Here's how the part is built. I have some questions about the finished solid (model axes, mm). Face numbers are marked on the shaded views. Give positions to 0.01 mm unless a question says otherwise; leave off trailing zeros. Put each result on its own line as item: value. Start each with the question number.
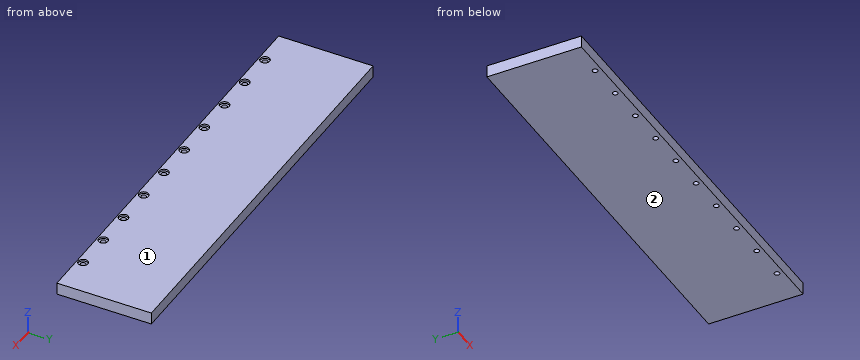
from build123d import *

# Parameters (mm, degrees)
SKETCH1_W                        = 220
SKETCH1_H                        = 50
BOSS_EXTRUDE1_DEPTH              = 3.175
CBORE_FOR_M2_5_SHCS1_D           = 2.7
CBORE_FOR_M2_5_SHCS1_DEPTH       = 15
CBORE_FOR_M2_5_SHCS1_CBORE_D     = 5
CBORE_FOR_M2_5_SHCS1_CBORE_DEPTH = 1
CBORE_FOR_M2_5_SHCS1_TIP         = 0.811161836


with BuildPart() as part:
    # Sketch1 → Boss-Extrude1 (new, symmetric)
    with BuildSketch(Plane.XY):
        Rectangle(SKETCH1_W, SKETCH1_H)
    extrude(amount=BOSS_EXTRUDE1_DEPTH, both=True)

    # CBORE for M2.5 SHCS1
    with Locations(Plane.XY.offset(3.175)):
        with Locations((89.95, -21.825), (69.9, -21.825), (49.85, -21.825), (29.8, -21.825), (9.75, -21.825), (-10.3, -21.825), (-30.35, -21.825), (-50.4, -21.825), (-70.45, -21.825), (-90.5, -21.825)):
            CounterBoreHole(CBORE_FOR_M2_5_SHCS1_D / 2, CBORE_FOR_M2_5_SHCS1_CBORE_D / 2, CBORE_FOR_M2_5_SHCS1_CBORE_DEPTH, depth=CBORE_FOR_M2_5_SHCS1_DEPTH)
            with Locations((0, 0, -(CBORE_FOR_M2_5_SHCS1_DEPTH + CBORE_FOR_M2_5_SHCS1_TIP / 2))):  # 118° drill point
                Cone(0, CBORE_FOR_M2_5_SHCS1_D / 2, CBORE_FOR_M2_5_SHCS1_TIP, mode=Mode.SUBTRACT)


solid = part.part
1) I'm going to push a flat-ended pin straight in: P1, Ø4.5, axis at x = -30.35, y = -21.825, coming from the +Z side (3 decimals). Where does the tip first touch, or does it pass through?
2) Thinking about a two-plate mould opening in Z: for the marked faces 1 and 2, which applies, pulls with the +Z half, pulls with the -Z half, needs draft (parallel to the pull), parting line crosses it, or undercut?
3) I need wall thicknesses on line 1 (Y direction, x = -50.4, z = 2.7) (3 decimals); line 2 (Y direction, x = 29.8, z = -0.9) (3 decimals). Which ranges of each line are inside material? Lowest first, please.
Ans:
1. P1: stops at z = 2.175
2. face 1: pulls with the +Z half
2. face 2: pulls with the -Z half
3. line 1: y = -25 to -24.325, -19.325 to 25
3. line 2: y = -25 to -23.175, -20.475 to 25
